```python
from build123d import *

# Parameters (mm, degrees)
ESQUISSE3_W                  = 364.4
ESQUISSE3_H                  = 85
ESQUISSE3_W_2                = 300
ESQUISSE3_H_2                = 62.7
ESQUISSE3_H_3                = 37.7
BOSS_EXTRU_1_DEPTH           = 10
ENL_V_MAT_EXTRU_1_DEPTH      = 10
ENL_V_MAT_EXTRU_2_DEPTH      = 211.627348652
ENL_V_MAT_EXTRU_2_DEPTH_BACK = 10
ESQUISSE10_R                 = 2.25
ESQUISSE10_R_2               = 3
ENL_V_MAT_EXTRU_3_DEPTH      = 10
ESQUISSE15_R                 = 2.25
ENL_V_MAT_EXTRU_4_DEPTH      = 10
CONG_1_R                     = 10
CONG_3_R                     = 1
ENL_V_MAT_EXTRU_5_DEPTH      = 10


with BuildPart() as part:
    # Esquisse3 → Boss.-Extru.1 (new body)
    with BuildSketch(Plane.XY):
        Rectangle(ESQUISSE3_W, ESQUISSE3_H)
        with Locations((0, 73.85)):
            Rectangle(ESQUISSE3_W_2, ESQUISSE3_H_2)
        with Locations((0, -61.35)):
            Rectangle(ESQUISSE3_W_2, ESQUISSE3_H_3)
        Polygon((-150, 105.2), (-182.2, 42.5), (-150, 42.5), align=None)
        Polygon((-150, -42.5), (-182.2, -42.5), (-150, -80.2), align=None)
        Polygon((182.2, -42.5), (150, -42.5), (150, -80.2), align=None)
        Polygon((182.2, 42.5), (150, 105.2), (150, 42.5), align=None)
    extrude(amount=BOSS_EXTRU_1_DEPTH)

    # Esquisse4 → Enlèv. mat.-Extru.1 (cut)
    with BuildSketch(Plane.XY.offset(10)):
        Polygon((-97.2, 32.5), (-122.2, 32.5), (-122.2, 22.5), (-182.2, 22.5), (-182.2, -22.5), (-122.2, -22.5), (-122.2, -32.5), (-97.2, -32.5), (-97.2, -37.5), (-62.2, -37.5), (-62.2, 37.5), (-97.2, 37.5), align=None)
        Polygon((122.2, 22.5), (122.2, 32.5), (97.2, 32.5), (97.2, 37.5), (62.2, 37.5), (62.2, -37.5), (97.2, -37.5), (97.2, -32.5), (122.2, -32.5), (122.2, -22.5), (182.2, -22.5), (182.2, 22.5), align=None)
    extrude(amount=-ENL_V_MAT_EXTRU_1_DEPTH, mode=Mode.SUBTRACT)

    # Esquisse5 → Enlèv. mat.-Extru.2 (cut, two sides: drawn at the far end of the back side and taken through both)
    with BuildSketch(Plane.XY.offset(10).offset(-ENL_V_MAT_EXTRU_2_DEPTH_BACK)):
        with BuildLine():
            Line((84.852813742, 105.2), (28.284271247, 105.2))
            ThreePointArc((28.284271247, 105.2), (56.568542495, 85.2), (84.852813742, 105.2))
        make_face()
        with BuildLine():
            ThreePointArc((-28.284271247, 105.2), (0, 85.2), (28.284271247, 105.2))
            Line((28.284271247, 105.2), (-28.284271247, 105.2))
        make_face()
        with BuildLine():
            ThreePointArc((-84.852813742, 105.2), (-56.568542495, 85.2), (-28.284271247, 105.2))
            Line((-28.284271247, 105.2), (-84.852813742, 105.2))
        make_face()
    extrude(amount=ENL_V_MAT_EXTRU_2_DEPTH + ENL_V_MAT_EXTRU_2_DEPTH_BACK, mode=Mode.SUBTRACT)

    # Esquisse10 → Enlèv. mat.-Extru.3 (cut)
    with BuildSketch(Plane.XY.offset(10)):
        with Locations((-147.7, 32.5)):
            Circle(ESQUISSE10_R)
        with Locations((-172.2, 32.5)):
            Circle(ESQUISSE10_R_2)
        with Locations((-172.2, -32.5)):
            Circle(ESQUISSE10_R_2)
        with Locations((-147.7, -32.5)):
            Circle(ESQUISSE10_R)
        with Locations((172.2, 32.5)):
            Circle(ESQUISSE10_R_2)
        with Locations((147.7, 32.5)):
            Circle(ESQUISSE10_R)
        with Locations((172.2, -32.5)):
            Circle(ESQUISSE10_R_2)
        with Locations((147.7, -32.5)):
            Circle(ESQUISSE10_R)
    extrude(amount=-ENL_V_MAT_EXTRU_3_DEPTH, mode=Mode.SUBTRACT)

    # Esquisse15 → Enlèv. mat.-Extru.4 (cut)
    with BuildSketch(Plane.XY.offset(10)):
        with Locations((-52.2, -23.2)):
            Circle(ESQUISSE15_R)
        with Locations((52.2, -23.2)):
            Circle(ESQUISSE15_R)
    extrude(amount=-ENL_V_MAT_EXTRU_4_DEPTH, mode=Mode.SUBTRACT)

    # Congé1
    cong_1_edges = [part.edges().sort_by_distance(p)[0] for p in [
        (150, -80.2, 5),
        (-150, -80.2, 5),
        (-150, 105.2, 5),
        (150, 105.2, 5),
    ]]
    fillet(cong_1_edges, radius=CONG_1_R)

    # Congé3
    cong_3_edges = [part.edges().sort_by_distance(p)[0] for p in [
        (-84.852813742, 105.2, 5),
        (84.852813742, 105.2, 5),
        (28.284271247, 105.2, 5),
        (-28.284271247, 105.2, 5),
    ]]
    fillet(cong_3_edges, radius=CONG_3_R)

    # Esquisse17 → Enlèv. mat.-Extru.5 (cut)
    with BuildSketch(Plane.XY.offset(10)):
        with BuildLine():
            Line((-40.31, 83.2), (-40.31, 73.2))
            ThreePointArc((-40.31, 73.2), (-42.81, 70.7), (-45.31, 73.2))
            Line((-45.31, 73.2), (-45.31, 83.2))
            ThreePointArc((-45.31, 83.2), (-42.81, 85.7), (-40.31, 83.2))
        make_face()
        with BuildLine():
            Line((-40.31, 65.2), (-40.31, 55.2))
            ThreePointArc((-40.31, 55.2), (-42.81, 52.7), (-45.31, 55.2))
            Line((-45.31, 55.2), (-45.31, 65.2))
            ThreePointArc((-45.31, 65.2), (-42.81, 67.7), (-40.31, 65.2))
        make_face()
    extrude(amount=-ENL_V_MAT_EXTRU_5_DEPTH, mode=Mode.SUBTRACT)


solid = part.part
```
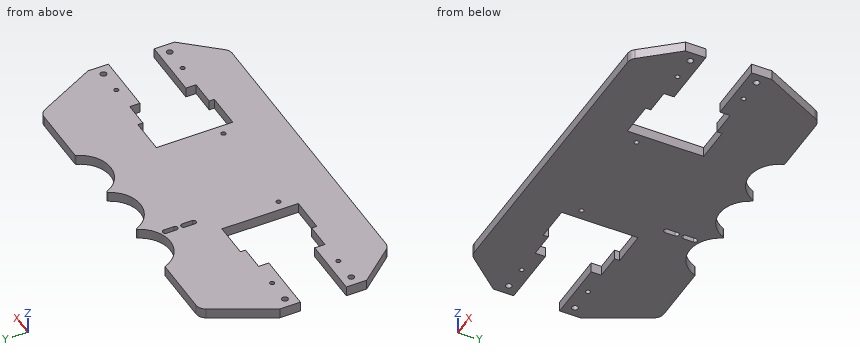
Source: CAD feature listing. Evaluate the final solid. Frame: model axes, mm. Round coordinates to 2 decimals unless told otherwise and drop trailing zeros. Write each loop counter-clockwise with the first axis right and the second up, starting at its lowest first coordinate (ties: lowest second). Pieces come first, ordered by that corner, then holes. Notation, with made-up numbers: M 0,-34.5 L 27,-34.5 A35 cw 27,-0.5 Z; hole C -26,-33 d5. An arc over 180 degrees is marked long. Answer as a JSON object with one key per item and string values. Group by question number.
(1) Ray query, line 1 (X direction, y = -36.5, z = 3.75); line 2 (Y direction, x = 172.2, z = 3); line 3 (Y direction, x = -147.7, z = 5.5). Return the intervals inside material, ascending. Write a range as [from, to].
(2) Section query C-C on y = 2. Output: boundary loops of the cut face in (x, z).
(3) Section query B-B on z = 2.25. State how many separate pieces and enclosed holes the cut face has, then the cut area to 3 significant figures.
(4) Section query A-A on x = 157. Output: boundary loops of the cut face in (y, z).
(5) Section query D-D on x = 72. Output: boundary loops of the cut face in (y, z).
(6) First-contact query: pin 1 (4 mm diameter, centred on x = -147.7, y = 32.5, fed in from +Z); pin 2 (2 mm diameter, centred on x = -31.5, z = 5.5, fed in from +Y). Flat tips, straight axial feed; report the tip coordinate or a pass-through.
Computed values:
{
 "1": {"line 1": "[-182.2, -97.2], [-62.2, 62.2], [97.2, 182.2]", "line 2": "[-54.21, -35.5], [-29.5, -22.5], [22.5, 29.5], [35.5, 61.97]", "line 3": "[-79.93, -34.75], [-30.25, -22.5], [22.5, 30.25], [34.75, 104.45]"},
 "2": {"outline": "M -62.2,0 L 62.2,0 L 62.2,10 L -62.2,10 Z"},
 "3": {"separate pieces": "1", "enclosed holes": "12", "area": "47,600 mm^2"},
 "4": {"outline": "M -72,0 L -22.5,0 L -22.5,10 L -72,10 Z; M 22.5,0 L 91.57,0 L 91.57,10 L 22.5,10 Z"},
 "5": {"outline": "M -80.2,0 L -37.5,0 L -37.5,10 L -80.2,10 Z; M 37.5,0 L 89.47,0 L 89.47,10 L 37.5,10 Z"},
 "6": {"pin 1": "through", "pin 2": "y = 100.35"}
}
